```python
from build123d import *

# Parameters (mm, degrees)
SKETCH1_R             = 19
MOTOR_MACHINERY_DEPTH = 60
SKETCH2_R             = 6
BOSS_EXTRUDE2_DEPTH   = 10
SKETCH5_R             = 3
MOTOR_SHAFT_DEPTH     = 20
SKETCH7_R             = 1
HUB_HOLES_DEPTH       = 20


with BuildPart() as part:
    # Sketch1 → motor machinery (new body)
    with BuildSketch(Plane.XY):
        Circle(SKETCH1_R)
    extrude(amount=MOTOR_MACHINERY_DEPTH)

    # Sketch2 → Boss-Extrude2 (add)
    with BuildSketch(Plane.XY.offset(60)):
        with Locations((2.459603008, 6.553651886)):
            Circle(SKETCH2_R)
    extrude(amount=BOSS_EXTRUDE2_DEPTH)

    # Sketch5 → motor shaft (add)
    with BuildSketch(Plane.XY.offset(70)):
        with Locations((2.459603008, 6.553651886)):
            Circle(SKETCH5_R)
    extrude(amount=MOTOR_SHAFT_DEPTH)

    # Sketch7 → hub holes (cut)
    with BuildSketch(Plane(origin=(0, 0, 0), x_dir=(1, 0, 0), z_dir=(0, 1, 0))):
        with Locations(Location((2.459603008, -80, 0), (0, 0, 90))):
            Circle(SKETCH7_R)
    extrude(amount=HUB_HOLES_DEPTH, mode=Mode.SUBTRACT)


solid = part.part
```
Source: CAD feature listing. Evaluate the final solid. Frame: model axes, mm. A direction names the side the tool comes from. Give positions to 0.01 mm unless a question says otherwise; leave off trailing zeros. Order: outer loops, then holes, each group sorted by start corner. A loop starts at its lowest first (then second) coordinate and runs counter-clockwise, first axis right, second up.
(1) Contact query for flat-ended pins moving along their axis: P1, Ø6, axis at y = -9, z = 58.5, coming from the +X side; P2, Ø1.5, axis at x = -2, y = -7, coming from the +Z side; P3, Ø3, axis at x = 2.46, z = 80, coming from the +Y side. Output: stop coordinate, or through.
(2) Section query A-A (z = 80). Return the cut outline in (x, y).
(3) Material intervals for line 1 along Z through (x, y) = (12.5, -9); line 2 along Z through (x, y) = (6, 9); line 3 along X through (y, z) = (5.75, 80), sorted ascending.
(4) Section query B-B (x = 4.5). Return the cut outline in (y, z), plus the area to 3 significant figures.
(5) Access query for faces 1 (the face through (5, 4, 70)), 2 (the face through (8.767, -16.856, 29.58)). Directions: +Z, -Z, +X, -X, +Y, -Y. A direction counts if a zero-diameter tool reaches every point of the face in a straight line with its end or side. Return the directions, or none.
(6) Section query D-D (z = 23.5). Return the cut outline in (x, y).
(7) Pull-direction query (X, two-part tool) for faces 3 (the face through (2.4, 6.5, 81)), 4 (the face through (0, 0, 0)), 5 (the face through (5.23, 5.4, 79.86)); classes: +X half, -X half, draft (parallel to the pull), parting line (faces both ways), or undercut.
(8) Section query C-C (y = 1.5). Return the cut outline in (x, z), plus the area to 3 significant figures.
Outcome:
1. P1: stops at x = 18.03
1. P2: stops at z = 60
1. P3: stops at y = 9.55
2. outline: (1.46, 3.73) - (1.46, 9.38) arc R3 ccw to start; (3.46, 3.73) arc R3 ccw to (3.46, 9.38) - close
3. line 1: z = 0 to 60
3. line 2: z = 0 to 70
3. line 3: x = -0.43 to 1.46, 3.46 to 5.35
4. outline: (-18.46, 0) - (18.46, 0) - (18.46, 60) - (12.2, 60) - (12.2, 70) - (8.75, 70) - (8.75, 90) - (4.35, 90) - (4.35, 70) - (0.91, 70) - (0.91, 60) - (-18.46, 60) - close
4. area: 2,420 mm2
5. face 1: +Z
5. face 2: +Z, -Z
6. outline: circle Ø38 at (0, 0)
7. face 3: undercut
7. face 4: draft
7. face 5: parting line
8. outline: (-18.94, 0) - (18.94, 0) - (18.94, 60) - (5.69, 60) - (5.69, 70) - (-0.77, 70) - (-0.77, 60) - (-18.94, 60) - close
8. area: 2,340 mm2
